```python
from build123d import *

# Parameters (mm, degrees)
F1_DEPTH = 80
F2_R     = 1.8
F3_DEPTH = 5.001
F4_SIZE  = 0.5
F5_SIZE  = 0.1


with BuildPart() as f1:
    # F0 (on Front) → F1 (new body)
    with BuildSketch(Plane.XZ):
        Polygon((0, 0.3), (0, 0), (15, 0), (15, 5), (5.219879, 5), align=None)
    extrude(amount=F1_DEPTH)

    # F2 (on face) → F3 (cut, through all)
    with BuildSketch(Plane.XY.offset(5)):
        with Locations((11, -40)):
            Circle(F2_R)
        with Locations((11, -15)):
            Circle(F2_R)
        with Locations((11, -65)):
            Circle(F2_R)
    extrude(amount=-F3_DEPTH, mode=Mode.SUBTRACT)

    # F4
    f4_edges = [f1.edges().sort_by_distance(p)[0] for p in [
        (15, -40, 0),
    ]]
    chamfer(f4_edges, length=F4_SIZE)

    # F5
    f5_edges = [f1.edges().sort_by_distance(p)[0] for p in [
        (15, -40, 5),
        (10.109939, -80, 5),
        (10.109939, 0, 5),
    ]]
    chamfer(f5_edges, length=F5_SIZE)


solid = f1.part
```
Model file for the job. Use its own axes, mm. Give positions to 0.01 mm unless a question says otherwise; leave off trailing zeros. Order: outer loops, then holes, each group sorted by start corner. A loop starts at its lowest first (then second) coordinate and runs counter-clockwise, first axis right, second up.
1) Mould opens along X. For faces 1 (the flat face through (3, -39, 3)), 2 (the flat face through (9, 0, 2)), 3 (the cylindrical face through (10.766, -38.215, 2.535)) say: +X half, -X half, draft (parallel to the pull), parting line (faces both ways), or undercut.
2) Saw through at B-B, the plane z = 3.7. Write the cut outline in (x, y).
3) Wall check: probe 1 along Y at (x, z) = (11, 3.7); probe 2 along X at (y, z) = (-65, 1.4); probe 3 along X at (y, z) = (-39, 4.55). Give the ranges that are in metal, low to high.
4) Saw through at C-C, the plane y = -19.5. Write the cut outline in (x, z), then the cut area to 3 significant figures.
5) Saw through at D-D, the plane x = 11.75. Write the cut outline in (y, z).
6) Saw through at A-A, the plane y = -40. Write the cut outline in (x, z).
Computed:
1. face 1: -X half
1. face 2: draft
1. face 3: undercut
2. outline: (3.78, -80) - (15, -80) - (15, 0) - (3.78, 0) - close; hole circle Ø3.6 at (11, -65); hole circle Ø3.6 at (11, -40); hole circle Ø3.6 at (11, -15)
3. probe 1: y = -80 to -66.8, -63.2 to -41.8, -38.2 to -16.8, -13.2 to 0
3. probe 2: x = 1.22 to 9.2, 12.8 to 15
3. probe 3: x = 4.72 to 9.5, 12.5 to 15
4. outline: (0, 0) - (14.5, 0) - (15, 0.5) - (15, 4.9) - (14.9, 5) - (5.22, 5) - (0, 0.3) - close
4. area: 62.6 mm2
5. outline: (-80, 0) - (-66.64, 0) - (-66.64, 5) - (-79.9, 5) - (-80, 4.9) - close; (-63.36, 0) - (-41.64, 0) - (-41.64, 5) - (-63.36, 5) - close; (-38.36, 0) - (-16.64, 0) - (-16.64, 5) - (-38.36, 5) - close; (-13.36, 0) - (0, 0) - (0, 4.9) - (-0.1, 5) - (-13.36, 5) - close
6. outline: (0, 0) - (9.2, 0) - (9.2, 5) - (5.22, 5) - (0, 0.3) - close; (12.8, 0) - (14.5, 0) - (15, 0.5) - (15, 4.9) - (14.9, 5) - (12.8, 5) - close
